Geometry check sheet. Reference: the model listing, model coordinates, mm. A direction names the side the tool comes from. Round coordinates to 2 decimals unless told otherwise and drop trailing zeros. Order: outer loops, then holes, each group sorted by start corner. A loop starts at its lowest first (then second) coordinate and runs counter-clockwise, first axis right, second up.
(1) Sectioned sample at C-C (y = 1.5). Record the boundary of the cut face in (x, z), plus the area to 3 significant figures.
(2) Sectioned sample at D-D (x = -5). Give the number of separate pieces and of enclosed holes in the cut face, plus the area to 3 significant figures.
(3) Go/stop test with flat-tipped pins: pin 1 (1.2 mm diameter, centred on x = 2, y = 7, fed in from -Z); pin 2 (5.5 mm diameter, centred on x = -5, z = 12, fed in from +Y); pin 3 (3 mm diameter, centred on x = -2, y = 4, fed in from +Z); pin 4 (3 mm diameter, centred on x = -5, z = -12, fed in from -Y). Record where each tip stops, or that it passes through.
(4) Material ranges on line 1 along Z through (x, y) = (-5, 1.2); line 2 along X through (y, z) = (1.05, -12); line 3 along Z through (x, y) = (-6.25, 4.5), recorded low to high.
(5) Release check for a two-part mould opening along X. For faces 1 (the face through (0, 7, 2.25)), 2 (the face through (-5.8, 1, 13.5)), 3 (the face through (-10.1, 1, 0)) record: +X half, -X half, draft (parallel to the pull), parting line (faces both ways), or undercut.
(6) Sectioned sample at A-A (z = 12). Record the boundary of the cut face in (x, y), plus the area to 3 significant figures.
(7) Sectioned sample at B-B (y = 3.5). Record the boundary of the cut face in (x, z).
(8) Set-up check for faces 4 (the face through (0.14, 5.51, -2.74)), 5 (the face through (0, 5, -7.25)), 6 (the face through (-0.141, 8.199, 2.535)): record each of +Z, -Z, +X, -X, +Y, -Y from which the full face is reachable in a straight line by a thin tool's end or side.
from build123d import *

# Parameters (mm, degrees)
SCHIZZO1_W                   = 20.2
SCHIZZO1_H                   = 34
ESTRUSIONE_ESTRUSIONE1_DEPTH = 2
ESTRUSIONE_ESTRUSIONE2_DEPTH = 20.2
SMUSSO1_SIZE                 = 1
RACCORDO2_R                  = 0.5
RACCORDO3_R                  = 1
FORO_PER_VITE_M3_1_D         = 3.4
SMUSSO1_OF_SPECCHIA2_SIZE    = 1
RACCORDO2_OF_SPECCHIA2_R     = 0.5
RACCORDO3_OF_SPECCHIA2_R     = 1


with BuildPart() as part:
    # Schizzo1 → Estrusione-Estrusione1 (new body)
    with BuildSketch(Plane(origin=(0, 0, 0), x_dir=(1, 0, 0), z_dir=(0, 1, 0))):
        Rectangle(SCHIZZO1_W, SCHIZZO1_H)
    extrude(amount=ESTRUSIONE_ESTRUSIONE1_DEPTH)

    # Schizzo3 → Estrusione-Estrusione2 (add)
    with BuildSketch(Plane(origin=(10.1, 0, 0), x_dir=(0, 0, -1), z_dir=(1, 0, 0))):
        Polygon((-7.25, 2), (-5.25, 2), (-5.25, 6), (-3.75, 6), (-3.75, 5), (-2.25, 5), (-2.25, 8.5), (-7.25, 8.5), align=None)
    estrusione_estrusione2 = extrude(amount=-ESTRUSIONE_ESTRUSIONE2_DEPTH)

    # Smusso1
    smusso1_edges = [part.edges().sort_by_distance(p)[0] for p in [
        (0, 5, 2.25),
    ]]
    chamfer(smusso1_edges, length=SMUSSO1_SIZE)

    # Raccordo2
    raccordo2_edges = [part.edges().sort_by_distance(p)[0] for p in [
        (0, 6, 5.25),
        (0, 6, 3.75),
    ]]
    fillet(raccordo2_edges, radius=RACCORDO2_R)
    raccordo2_2_edges = [part.edges().sort_by_distance(p)[0] for p in [
        (0, 8.5, 7.25),
        (0, 5, 3.75),
    ]]
    fillet(raccordo2_2_edges, radius=RACCORDO2_R - 0.0001)  # a hair under: the kernel refuses the full size

    # Raccordo3
    raccordo3_edges = [part.edges().sort_by_distance(p)[0] for p in [
        (0, 8.5, 2.25),
    ]]
    fillet(raccordo3_edges, radius=RACCORDO3_R)

    # Foro per Vite M3-1 (through all)
    with Locations(Plane(origin=(0, 2, 0), x_dir=(1, 0, 0), z_dir=(0, 1, 0))):
        with Locations((-5, -12), (5, -12)):
            foro_per_vite_m3_1 = Hole(FORO_PER_VITE_M3_1_D / 2)

    # Specchia2: Estrusione-Estrusione2, Foro per Vite M3-1 across plane
    add(estrusione_estrusione2.mirror(Plane.XY))
    add(foro_per_vite_m3_1.mirror(Plane.XY), mode=Mode.SUBTRACT)

    # Smusso1 of Specchia2
    smusso1_of_specchia2_edges = [part.edges().sort_by_distance(p)[0] for p in [
        (0, 5, -2.25),
    ]]
    chamfer(smusso1_of_specchia2_edges, length=SMUSSO1_OF_SPECCHIA2_SIZE)

    # Raccordo2 of Specchia2
    raccordo2_of_specchia2_edges = [part.edges().sort_by_distance(p)[0] for p in [
        (0, 6, -5.25),
        (0, 6, -3.75),
    ]]
    fillet(raccordo2_of_specchia2_edges, radius=RACCORDO2_OF_SPECCHIA2_R)
    raccordo2_of_specchia2_2_edges = [part.edges().sort_by_distance(p)[0] for p in [
        (0, 8.5, -7.25),
        (0, 5, -3.75),
    ]]
    fillet(raccordo2_of_specchia2_2_edges, radius=RACCORDO2_OF_SPECCHIA2_R - 0.0001)  # a hair under: the kernel refuses the full size

    # Raccordo3 of Specchia2
    raccordo3_of_specchia2_edges = [part.edges().sort_by_distance(p)[0] for p in [
        (0, 8.5, -2.25),
    ]]
    fillet(raccordo3_of_specchia2_edges, radius=RACCORDO3_OF_SPECCHIA2_R)


solid = part.part
Answer below:
1. outline: (-10.1, -17) - (10.1, -17) - (10.1, 17) - (-10.1, 17) - close; hole circle Ø3.4 at (-5, -12); hole circle Ø3.4 at (-5, 12); hole circle Ø3.4 at (5, -12); hole circle Ø3.4 at (5, 12)
1. area: 650 mm2
2. separate pieces: 3
2. enclosed holes: 0
2. area: 97.0 mm2
3. pin 1: stops at z = -7.25
3. pin 2: stops at y = 2
3. pin 3: stops at z = 7.25
3. pin 4: passes through
4. line 1: z = -17 to -13.7, -10.3 to 10.3, 13.7 to 17
4. line 2: x = -10.1 to -6.7, -3.3 to 3.3, 6.7 to 10.1
4. line 3: z = -7.25 to -5.25, 5.25 to 7.25
5. face 1: draft
5. face 2: undercut
5. face 3: -X half
6. outline: (-10.1, 0) - (-6.7, 0) - (-6.7, 2) - (-10.1, 2) - close; (-3.3, 0) - (3.3, 0) - (3.3, 2) - (-3.3, 2) - close; (6.7, 0) - (10.1, 0) - (10.1, 2) - (6.7, 2) - close
6. area: 26.8 mm2
7. outline: (-10.1, -7.25) - (10.1, -7.25) - (10.1, -5.25) - (-10.1, -5.25) - close; (-10.1, 5.25) - (10.1, 5.25) - (10.1, 7.25) - (-10.1, 7.25) - close
8. face 4: +X, -X
8. face 5: -Z, +X, -X, +Y
8. face 6: +X, -X, +Y
